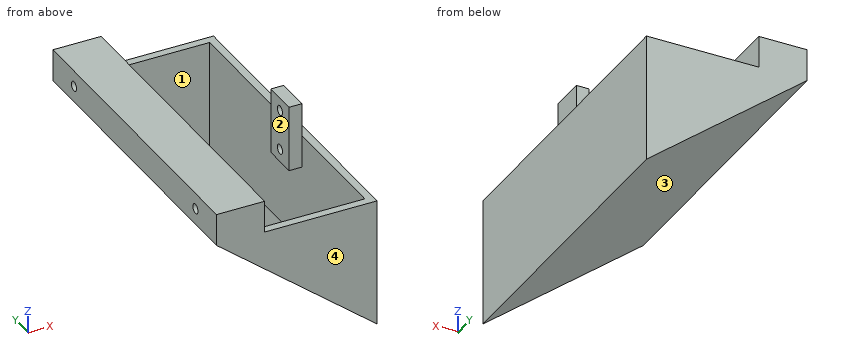
Autodesk Inventor part; units mm, degrees
ref_plane "YZ Plane" through (0, 0, 0) normal (1, 0, 0) x (0, 1, 0)
ref_plane "XZ Plane" through (0, 0, 0) normal (0, 1, 0) x (-1, 0, 0)
ref_plane "XY Plane" through (0, 0, 0) normal (0, 0, 1) x (1, 0, 0)
sketch "Esboço1" plane through (0, 0, 0) normal (0, 1, 0) x (-1, 0, 0)
  line L0 (0, 20) -> (0, -20)
  line L1 (0, 20) -> (50, 20)
  line L2 (50, 20) -> (0, -20)
  line L3 (50, 20) -> (50, 30)
  line L4 (50, 30) -> (35, 30)
  line L5 (35, 30) -> (35, 20)
  point P0 (0, 0)
  dimension "d0" = 40
  dimension "d1" = 50
  dimension "d2" = 10
  dimension "d3" = 15
extrude "Extrusão1" add sketch "Esboço1" along normal blind 97.084
shell "Casca1" thickness 2.5 removed faces 1 at (-23.3333, 32.3613, 20)
sketch "Esboço2" plane through (-50, 0, 20) normal (-1, 0, 0) x (0, 0, 1)
  line L0 (10, 97.084) -> (0, 97.084)
  line L1 (0, 97.084) -> (5, 97.084)
  line L2 (5, 97.084) -> (5, 84.584)
  circle A0 centre (5, 84.584) radius 1.5
  line L3 (10, 0) -> (0, 0)
  line L4 (0, 0) -> (5, 0)
  line L5 (5, 0) -> (5, 12.5)
  circle A1 centre (5, 12.5) radius 1.5
  point P0 (-20, 0)
  dimension "d7" = 5
  dimension "d8" = 12.5
  dimension "d9" = 3
  dimension "d10" = 5
  dimension "d11" = 12.5
  dimension "d12" = 3
extrude "Extrusão2" cut sketch "Esboço2" against normal blind 102.84
thread "Rosca1"
thread "Rosca2"
thread "Rosca3"
thread "Rosca4"
sketch "Esboço3" plane through (0, 97.084, 0) normal (0, 1, 0) x (1, 0, 0)
  line L0 (-50, -30) -> (-35, -30)
  point P0 (0, 0)
  point P1 (-35, -20)
  dimension "d23" = 10
sketch "Esboço4" plane through (-50, 0, 20) normal (-1, 0, 0) x (0, 0, 1)
  line L0 (0, 97.084) -> (10, 97.084)
  line L1 (0, 0) -> (10, 0)
  point P0 (-20, 0)
  dimension "d24" = 97.084
sketch "Esboço5" plane through (0, 97.084, 0) normal (0, 1, 0) x (1, 0, 0)
  point P0 (0, 0)
sketch "Esboço6" plane through (-2.5, 2.5, 20) normal (-1, 0, 0) x (0, 0, 1)
  line L0 (-10.2933, 37.3647) -> (10.2933, 37.3647)
  line L1 (10.2933, 37.3647) -> (10.2933, 48.1592)
  line L2 (10.2933, 48.1592) -> (-10.2933, 48.1592)
  line L3 (-10.2933, 48.1592) -> (-10.2933, 37.3647)
  line L4 (0, 92.084) -> (0, 0)
  line L5 (-10.2933, 37.3647) -> (10.2933, 48.1592) construction
  line L6 (10.2933, 37.3647) -> (-10.2933, 48.1592) construction
  point P0 (-20, -2.5)
  point P1 (0, 42.762)
extrude "Extrusão3" add sketch "Esboço6" along normal blind 4
sketch "Esboço7" plane through (-6.5, 2.5, 20) normal (-1, 0, 0) x (0, 0, 1)
  line L0 (-10.2933, 48.1592) -> (-10.2933, 37.3647)
  line L1 (-10.2933, 42.762) -> (-6.2933, 42.762)
  line L2 (10.2933, 37.3647) -> (10.2933, 48.1592)
  line L3 (10.2933, 42.762) -> (6.2933, 42.762)
  circle A0 centre (-6.2933, 42.762) radius 1.5
  circle A1 centre (6.2933, 42.762) radius 1.5
  point P0 (-20, -2.5)
  dimension "d27" = 4
  dimension "d28" = 4
  dimension "d29" = 3
  dimension "d30" = 3
extrude "Extrusão4" cut sketch "Esboço7" against normal blind 3.5
thread "Rosca5"
thread "Rosca6"
properties part number "Rampa 1"
For this review, take the finished solid that the model builds, in its own axes (mm). Face numbers are marked on the shaded views. Give positions to 0.01 mm unless a question says otherwise; leave off trailing zeros. Loops run counter-clockwise (first coordinate to the right, second up) from the corner with the lowest first, then second, coordinate; pieces in that order, holes last.
Item 1: Take a section at B-B, the plane y = 41.5. State the section outline as (x, z) points, and give its area (3 significant figures).
Item 2: Take a section at D-D, the plane x = -17. State the section outline as (y, z) points, and give its area (3 significant figures).
Item 3: Take a section at C-C, the plane x = -38.5. State the section outline as (y, z) points.
Item 4: Draft analysis for pull direction X (two halves, no side actions). For the marked faces 1, 2, 3 and 4, state which applies: +X half, -X half, draft (parallel to the pull), parting line (faces both ways), or undercut.
Item 5: For line 1 along Y through (x, z) = (-48.9, 25); line 2 along X through (y, z) = (23.5, 26); line 3 along Y through (x, z) = (-8, -5), list the stretches that pass through material, from the lowest coordinate up.
Item 6: Take a section at A-A, the plane y = 12.5. State the section outline as (x, z) points.
Item 7: Insertion check: pin 1 (3 mm diameter, centred on x = -36, y = 46.5, fed in from -Z); pin 2 (2 mm diameter, centred on x = -4.5, y = 44.5, fed in from -Z); pin 3 (5 mm diameter, centred on x = -14, y = 66.5, fed in from +Z). Each pin has a flat end and moves straight along its axis. Give the tip position at first contact, or say it passes through.
Calculated:
1. outline: (-50, 20) - (0, -20) - (0, 20) - (-2.5, 20) - (-2.5, 30.29) - (-6.5, 30.29) - (-6.5, 9.71) - (-2.5, 9.71) - (-2.5, -14.8) - (-47.5, 21.2) - (-47.5, 27.5) - (-37.5, 27.5) - (-37.5, 20) - (-35, 20) - (-35, 30) - (-50, 30) - close
1. area: 401 mm2
2. outline: (0, -6.4) - (97.08, -6.4) - (97.08, 20) - (94.58, 20) - (94.58, -3.2) - (2.5, -3.2) - (2.5, 20) - (0, 20) - close
2. area: 427 mm2
3. outline: (0, 10.8) - (97.08, 10.8) - (97.08, 30) - (0, 30) - close; hole (2.5, 14) - (94.58, 14) - (94.58, 27.5) - (2.5, 27.5) - close
4. face 1: undercut
4. face 2: undercut
4. face 3: -X half
4. face 4: draft
5. line 1: y = 0 to 11, 14 to 83.08, 86.08 to 97.08
5. line 2: x = -50 to -47.5, -37.5 to -35
5. line 3: y = 0 to 2.5, 94.58 to 97.08
6. outline: (-50, 20) - (0, -20) - (0, 20) - (-2.5, 20) - (-2.5, -14.8) - (-47.5, 21.2) - (-47.5, 23.5) - (-50, 23.5) - close; (-50, 26.5) - (-47.5, 26.5) - (-47.5, 27.5) - (-37.5, 27.5) - (-37.5, 26.5) - (-35, 26.5) - (-35, 30) - (-50, 30) - close; (-37.5, 20) - (-35, 20) - (-35, 23.5) - (-37.5, 23.5) - close
7. pin 1: stops at z = 7.6
7. pin 2: stops at z = -17.2
7. pin 3: stops at z = -3.6
